Check sheet for the modelled part. Datum: model origin and axes. Units: mm. Face numbers are marked on the shaded views. Give positions to 0.01 mm unless a question says otherwise; leave off trailing zeros.
from build123d import *

# Parameters (mm, degrees)
SKETCH1_R          = 20
EXTRUDE1_DEPTH     = 40
SKETCH2_R          = 2.5
SKETCH4_R          = 18
CUT_EXTRUDE1_DEPTH = 38
FILLET1_R          = 0.75
FILLET2_R          = 0.75
SCALE2_SCALE       = 1.8


with BuildPart() as part:
    # Sketch1 → Extrude1 (new body)
    with BuildSketch(Plane(origin=(0, 0, 0), x_dir=(1, 0, 0), z_dir=(0, 1, 0))):
        Circle(SKETCH1_R)
    extrude(amount=EXTRUDE1_DEPTH)

    # Sweep1: sweep along a path in Sketch3
    with BuildLine(Plane.XY) as sweep1_path:
        Line((0, 30.773001508), (21.65, 30.773001508))
        ThreePointArc((21.65, 30.773001508), (33.01, 19.413001508), (21.65, 8.053001508))
        Line((21.65, 8.053001508), (0, 8.053001508))
    # Sketch2 → Sweep1 (sweep)
    with BuildSketch(Plane(origin=(0, 0, 0), x_dir=(0, 0, -1), z_dir=(1, 0, 0))):
        with Locations((0, 33.273001508)):
            Circle(SKETCH2_R)
    sweep(path=sweep1_path.line)

    # Sketch4 → Cut-Extrude1 (cut)
    with BuildSketch(Plane(origin=(0, 40, 0), x_dir=(-1, 0, 0), z_dir=(0, 1, 0))):
        Circle(SKETCH4_R)
    extrude(amount=-CUT_EXTRUDE1_DEPTH, mode=Mode.SUBTRACT)

    # Fillet1
    fillet1_edges = [part.edges().sort_by_distance(p)[0] for p in [
        (18, 40, 0),
        (-20, 40, 0),
    ]]
    fillet(fillet1_edges, radius=FILLET1_R)

    # Fillet2
    fillet2_edges = [part.edges().sort_by_distance(p)[0] for p in [
        (18, 2, 0),
    ]]
    fillet(fillet2_edges, radius=FILLET2_R)


with BuildPart() as part_1:
    # Scale2: scaled about (2.200885097, 16.795438051, 2.029e-06)
    add(part.part.scale(SCALE2_SCALE).moved(Location((-1.760708078, -13.436350441, -1.623e-06))))


solid = part_1.part
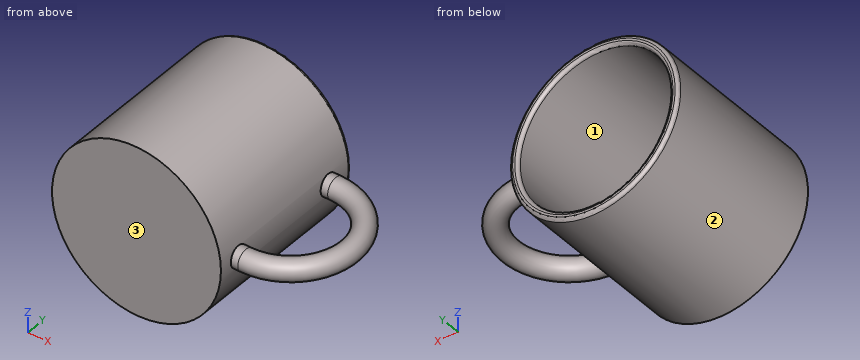
1) Draft check along Z on the marked faces 1, 2 and 3. Enter one of: +Z half, -Z half, draft (parallel to the pull), parting line (faces both ways), or undercut.
Recorded:
face 1: undercut
face 2: parting line
face 3: draft
2) Depth check by flat-ended pin: pin 1 Ø1 at (y, z) = (48.5, 24.5) entering from +X; pin 2 Ø2 at (y, z) = (21.5, 21.5) entering from -X; pin 3 Ø6 at (x, y) = (7, 21.5) entering from -Z. Enter the tip coordinate at first touch or a pass-through.
Recorded:
pin 1: stops at x = 25.07
pin 2: stops at x = -31.35
pin 3: stops at z = -35.54
3) Material ranges on L1, parallel to Z at x = -3, y = -5.5; L2, parallel to Y at x = 3.5, z = 30; L3, parallel to X at y = 3, z = -11, recorded low to high.
Recorded:
L1: z = -35.98 to -32.38, 32.38 to 35.98
L2: y = -13.44 to -9.84
L3: x = -36.04 to -32.24, 28.71 to 32.52
4) Section check A-A, the plane y = 9. State how many separate pieces and enclosed holes the cut face has, then the cut area to 3 significant figures.
Recorded:
separate pieces: 2
enclosed holes: 1
area: 848 mm2
